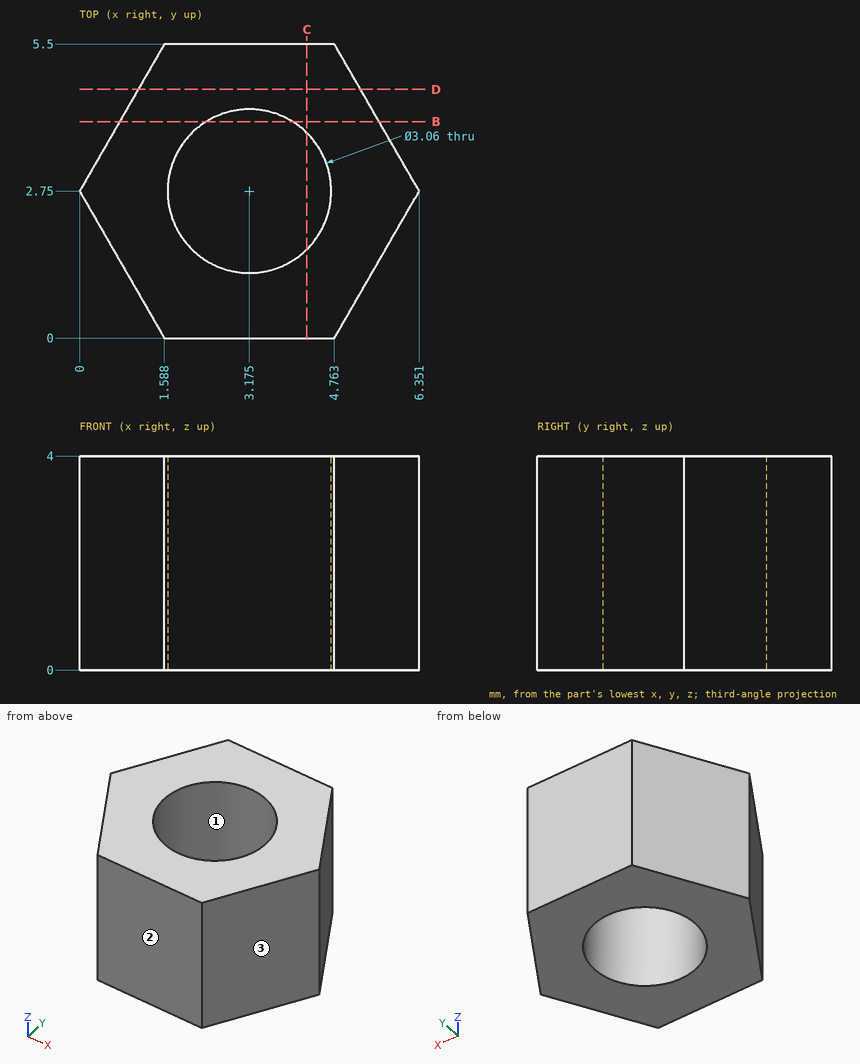
Verification items for this drawing (mm, ordinates from the low corner). Coordinates: 2 decimals unless noted, no trailing zeros. Write each loop counter-clockwise with the first axis right and the second up, starting at its lowest first coordinate (ties: lowest second). Pieces come first, ordered by that corner, then holes. Notation, with made-up numbers: M -3,51.25 L 9,51.25 A21 ccw 9,57.25 Z; hole C 34.25,32.25 d3. An arc over 180 degrees is marked long. Answer as CSV lines item,"result".
Q1. Cross-section at C-C (x = 4.25). Record the boundary of the cut face in (y, z), then the cut area to 3 significant figures.
Check result:
outline,"M 0,0 L 1.66,0 L 1.66,4 L 0,4 Z; M 3.84,0 L 5.5,0 L 5.5,4 L 3.84,4 Z"
area,"13.3 mm^2"
Q2. Material ranges on probe 1 along X at (y, z) = (4.15, 2.35) (1 decimal); probe 2 along X at (y, z) = (3, 3.4) (1 decimal); probe 3 along Y at (x, z) = (2.25, 2.2), recorded low to high. Write a range as from..to.
Check result:
probe 1,"0.8..2.6, 3.8..5.5"
probe 2,"0.1..1.7, 4.7..6.2"
probe 3,"0..1.53, 3.97..5.5"
Q3. Go/stop test with a flat-tipped pin: pin 1 (2 mm diameter, centred on x = 1.5, y = 2.5, fed in from -Z). Record where the tip stops, or that it passes through.
Check result:
pin 1,"z = 0"
Q4. Cross-section at B-B (y = 4.05). Record the boundary of the cut face in (x, z).
Check result:
outline,"M 0.75,0 L 2.37,0 L 2.37,4 L 0.75,4 Z; M 3.98,0 L 5.6,0 L 5.6,4 L 3.98,4 Z"
Q5. Cross-section at D-D (y = 4.65). Record the boundary of the cut face in (x, z), then the cut area to 3 significant figures.
Check result:
outline,"M 1.1,0 L 5.25,0 L 5.25,4 L 1.1,4 Z"
area,"16.6 mm^2"
Q6. Mould release check, pull along X, two halves, no side actions. Record for the marked faces 1, 2 and 3: released by +X, released by -X, zero draft, split by the parting line, or undercut.
Check result:
face 1,"undercut"
face 2,"zero draft"
face 3,"released by +X"
